from build123d import *

# Parameters (mm, degrees)
SKETCH1_R               = 10.85
SKETCH1_R_2             = 8.45
BOSS_EXTRUDE1_DEPTH     = 151.72
SKETCH3_R               = 2
CUT_EXTRUDE2_DEPTH      = 153.493945454
CUT_EXTRUDE3_DEPTH      = 153.493945567
CUT_EXTRUDE3_DEPTH_BACK = 153.493945567
SKETCH4_R               = 2


with BuildPart() as part:
    # Sketch1 → Boss-Extrude1 (new body)
    with BuildSketch(Plane(origin=(0, 0, 0), x_dir=(1, 0, 0), z_dir=(0, 1, 0))):
        with Locations(Location((0, 0, 0), (0, 0, 270))):
            Circle(SKETCH1_R)
        with Locations(Location((0, 0, 0), (0, 0, 270))):
            Circle(SKETCH1_R_2, mode=Mode.SUBTRACT)
    extrude(amount=BOSS_EXTRUDE1_DEPTH)

    # Sketch3 → Cut-Extrude2 (cut, through all)
    with BuildSketch(Plane.XY):
        with Locations(Location((0, 9.28, 0), (0, 0, 90))):
            Circle(SKETCH3_R)
    extrude(amount=-CUT_EXTRUDE2_DEPTH, mode=Mode.SUBTRACT)

    # Sketch4 → Cut-Extrude3 (cut, two sides: drawn at the far end of the back side and taken through both)
    with BuildSketch(Plane(origin=(0, 0, 0), x_dir=(0, 0, -1), z_dir=(1, 0, 0)).offset(-CUT_EXTRUDE3_DEPTH_BACK)):
        with Locations((0, 9.28)):
            Circle(SKETCH4_R)
    extrude(amount=CUT_EXTRUDE3_DEPTH + CUT_EXTRUDE3_DEPTH_BACK, mode=Mode.SUBTRACT)


solid = part.part
Source: CAD feature listing. Evaluate the final solid. Frame: model axes, mm. Round coordinates to 2 decimals unless told otherwise and drop trailing zeros. Loops run counter-clockwise (first coordinate to the right, second up) from the corner with the lowest first, then second, coordinate; pieces in that order, holes last. Notation, with made-up numbers: (86, 44.5) - (124, 44.5) arc R25 ccw to (124, 79.5) - close; hole circle Ø2 at (4, 77.25). An arc over 180 degrees is marked (long way). Write item = value, one per line. Start each with the question number.
Item 1: Section query D-D on y = 83.5. Output: boundary loops of the cut face in (x, z).
Item 2: Section query B-B on z = 0. Output: boundary loops of the cut face in (x, y).
Item 3: Mould query, pull axis X, two halves, no side actions, for faces 1 (the face through (3.26, 74.8, 10.35)), 2 (the face through (0.766, 11.127, -9.511)), 3 (the face through (2.54, 74.8, 8.06)), 4 (the face through (-9.548, 9.368, 1.998)). Classes: released by +X, released by -X, zero draft, split by the parting line, or undercut.
Item 4: Material intervals for line 1 (Y direction, x = 9.2, z = 0); line 2 (Z direction, x = -0.5, y = 37.5); line 3 (Z direction, x = -4.75, y = 108) (3 decimals), sorted ascending.
Item 5: First-contact query: pin 1 Ø3 at (x, y) = (0, 9.28) entering from -Z; pin 2 Ø12 at (x, y) = (2, 66) entering from -Z; pin 3 Ø1.5 at (x, y) = (-8.5, 94) entering from +Z; pin 4 Ø2 at (y, z) = (40.5, 7) entering from +X. Flat tips, straight axial feed; report the tip coordinate or a pass-through.
Item 6: Section query C-C on z = -6.75. Output: boundary loops of the cut face in (x, y), plus the area to 3 significant figures.
Item 7: Section query A-A on x = 0. Output: boundary loops of the cut face in (y, z).
Results list:
q1.outline = circle Ø21.7 at (0, 0); hole circle Ø16.9 at (0, 0)
q2.outline = (-10.85, 0) - (-8.45, 0) - (-8.45, 7.28) - (-10.85, 7.28) - close; (-10.85, 11.28) - (-8.45, 11.28) - (-8.45, 151.72) - (-10.85, 151.72) - close; (8.45, 0) - (10.85, 0) - (10.85, 7.28) - (8.45, 7.28) - close; (8.45, 11.28) - (10.85, 11.28) - (10.85, 151.72) - (8.45, 151.72) - close
q3.face_1 = split by the parting line
q3.face_2 = undercut
q3.face_3 = undercut
q3.face_4 = zero draft
q4.line_1 = 0 to 7.28, 11.28 to 151.72
q4.line_2 = -10.84 to -8.44, 8.44 to 10.84
q4.line_3 = -9.755 to -6.989, 6.989 to 9.755
q5.pin_1 = 8.32
q5.pin_2 = -10.85
q5.pin_3 = 7.59
q5.pin_4 = 9.04
q6.outline = (-8.49, 0) - (-5.08, 0) - (-5.08, 151.72) - (-8.49, 151.72) - close; (5.08, 0) - (8.49, 0) - (8.49, 151.72) - (5.08, 151.72) - close
q6.area = 1,040 mm²
q7.outline = (0, -10.85) - (7.28, -10.85) - (7.28, -8.45) - (0, -8.45) - close; (0, 8.45) - (151.72, 8.45) - (151.72, 10.85) - (0, 10.85) - close; (11.28, -10.85) - (151.72, -10.85) - (151.72, -8.45) - (11.28, -8.45) - close
